Answer from the drawing. Dimensions are ordinates in mm from the lowest x, y and z of the part. A direction names the side the tool comes from. Coordinates: 2 decimals unless noted, no trailing zeros. Write each loop counter-clockwise with the first axis right and the second up, starting at its lowest first coordinate (ties: lowest second). Pieces come first, ordered by that corner, then holes. Notation, with made-up numbers: (14.25, -6) - (65.25, -6) arc R17 ccw to (65.25, 7) - close; hole circle Ø9 at (6.25, 17). An arc over 180 degrees is marked (long way). Return JSON: item names as keys, results as strings.
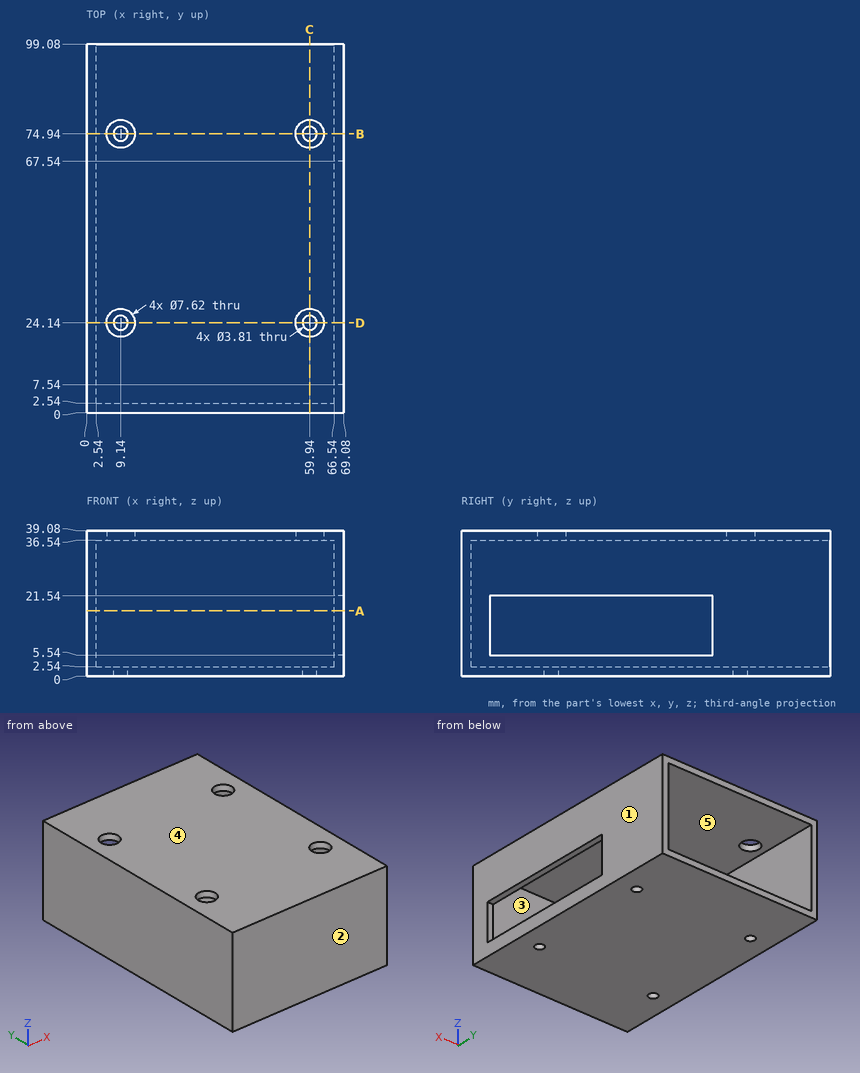
(1) Determine the mould class of the marked faces 1, 2 and 3 for opening direction X: +X half, -X half, draft (parallel to the pull), parting line (faces both ways), or undercut.
Answer:
{"face 1": "+X half", "face 2": "draft", "face 3": "undercut"}
(2) A cutting plane is placed at D-D (y = 24.14). Determine the outline of the cut face in (x, z) (3 decimals).
Answer:
{"outline": "(0, 0) - (7.235, 0) - (7.235, 2.54) - (2.54, 2.54) - (2.54, 36.54) - (5.33, 36.54) - (5.33, 39.08) - (0, 39.08) - close; (11.045, 0) - (58.035, 0) - (58.035, 2.54) - (11.045, 2.54) - close; (12.95, 36.54) - (56.13, 36.54) - (56.13, 39.08) - (12.95, 39.08) - close; (61.845, 0) - (69.08, 0) - (69.08, 5.54) - (66.54, 5.54) - (66.54, 2.54) - (61.845, 2.54) - close; (63.75, 36.54) - (66.54, 36.54) - (66.54, 21.54) - (69.08, 21.54) - (69.08, 39.08) - (63.75, 39.08) - close"}
(3) A cutting plane is placed at B-B (y = 74.94). Determine the outline of the cut face in (x, z) (3 decimals).
Answer:
{"outline": "(0, 0) - (7.235, 0) - (7.235, 2.54) - (2.54, 2.54) - (2.54, 36.54) - (5.33, 36.54) - (5.33, 39.08) - (0, 39.08) - close; (11.045, 0) - (58.035, 0) - (58.035, 2.54) - (11.045, 2.54) - close; (12.95, 36.54) - (56.13, 36.54) - (56.13, 39.08) - (12.95, 39.08) - close; (61.845, 0) - (69.08, 0) - (69.08, 39.08) - (63.75, 39.08) - (63.75, 36.54) - (66.54, 36.54) - (66.54, 2.54) - (61.845, 2.54) - close"}
(4) Flat-ended cylindrical pins translate along their axes: P1, Ø4.5, axis at x = 59.94, y = 74.94, coming from the -Z side; P2, Ø3, axis at x = 10, z = 23, coming from the +Y side. Find the tip coordinate at first contact, or state that the pin passes through.
Answer:
{"P1": "z = 0", "P2": "y = 2.54"}
(5) Which of the six approach directions +Z, -Z, +X, -X, +Y, -Y give full straight-line access (tool end or side, diameter ignored) to the marked faces 4 and 5?
Answer:
{"face 4": "+Z, +X, -X, +Y, -Y", "face 5": "+Y"}
(6) A cutting plane is placed at A-A (z = 17.5). Determine the outline of the cut face in (x, y), and give its area (3 significant figures).
Answer:
{"outline": "(0, 0) - (69.08, 0) - (69.08, 7.54) - (66.54, 7.54) - (66.54, 2.54) - (2.54, 2.54) - (2.54, 99.08) - (0, 99.08) - close; (66.54, 67.54) - (69.08, 67.54) - (69.08, 99.08) - (66.54, 99.08) - close", "area": "513 mm²"}
(7) A cutting plane is placed at C-C (x = 59.94). Determine the outline of the cut face in (y, z) (3 decimals).
Answer:
{"outline": "(0, 0) - (22.235, 0) - (22.235, 2.54) - (2.54, 2.54) - (2.54, 36.54) - (20.33, 36.54) - (20.33, 39.08) - (0, 39.08) - close; (26.045, 0) - (73.035, 0) - (73.035, 2.54) - (26.045, 2.54) - close; (27.95, 36.54) - (71.13, 36.54) - (71.13, 39.08) - (27.95, 39.08) - close; (76.845, 0) - (99.08, 0) - (99.08, 2.54) - (76.845, 2.54) - close; (78.75, 36.54) - (99.08, 36.54) - (99.08, 39.08) - (78.75, 39.08) - close"}
(8) Straight lines are drawn through the part: line 1 (X direction, y = 24.14, z = 37.45); line 2 (Y direction, x = 59.94, z = 37.25); line 3 (Y direction, x = 9, z = 1). For each, find the intervals that lie inside material, in ascending order. Write a range as from..to.
Answer:
{"line 1": "0..5.33, 12.95..56.13, 63.75..69.08", "line 2": "0..20.33, 27.95..71.13, 78.75..99.08", "line 3": "0..22.24, 26.04..73.04, 76.84..99.08"}
